Check sheet for the drawn part. Datum: minimum x, y, z corner. Units: mm. A direction names the side the tool comes from. Round coordinates to 2 decimals unless told otherwise and drop trailing zeros. Order: outer loops, then holes, each group sorted by start corner. A loop starts at its lowest first (then second) coordinate and runs counter-clockwise, first axis right, second up. Notation, with made-up numbers: (1.25, 1) -> (9.25, 1) arc R15 ccw to (9.25, 13) -> close; hole circle Ø2 at (34.5, 82). An arc over 180 degrees is marked (long way). Answer in a Markdown table with one row per item.
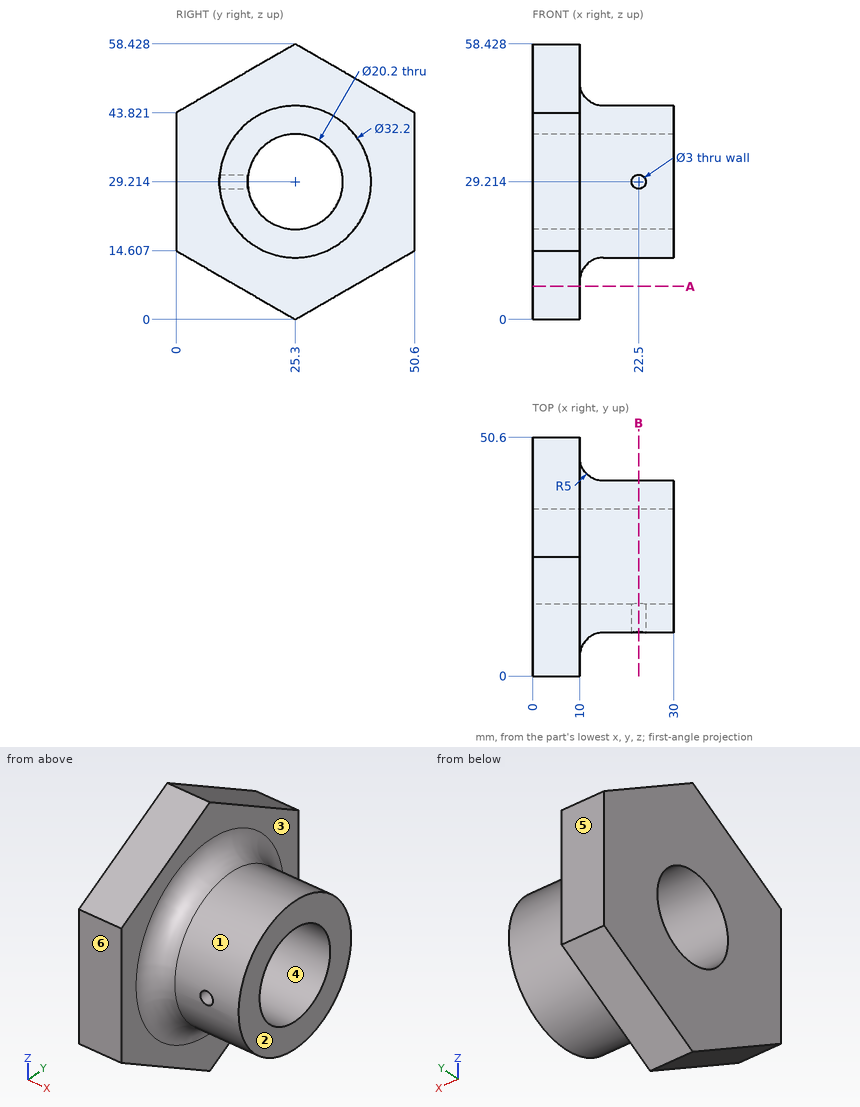
(1) Scan lines: probe 1 along Y at (x, z) = (22, 20.5); probe 2 along X at (y, z) = (36, 50); probe 3 along Y at (x, z) = (9, 36). Record each from-to range of solid material in increasing order. Write a range as from..to.
Solutions:
| item | result |
|---|---|
| probe 1 | 11.76..20.19, 30.41..38.84 |
| probe 2 | 0..10 |
| probe 3 | 0..17.82, 32.78..50.6 |
(2) Tool access check on the marked faces 1 and 2. Record the directions out of +Z, -Z, +X, -X, +Y, -Y that give a thin tool (end or side, any length) a straight path to the whole face; none if there is none.
Solutions:
| item | result |
|---|---|
| face 1 | +X |
| face 2 | +Z, -Z, +X, +Y, -Y |
(3) Draft check along Y on the marked faces 3, 4, 5 and 6. Enter one of: pulls with the +Y half, pulls with the -Y half, needs draft (parallel to the pull), parting line crosses it, or undercut.
Solutions:
| item | result |
|---|---|
| face 3 | needs draft |
| face 4 | undercut |
| face 5 | pulls with the +Y half |
| face 6 | pulls with the -Y half |
(4) Section check A-A on z = 7. Record the boundary of the cut face in (x, y), plus the area to 4 significant figures.
Solutions:
| item | result |
|---|---|
| outline | (0, 13.18) -> (10, 13.18) -> (10, 37.42) -> (0, 37.42) -> close |
| area | 242.5 mm^2 |
(5) Depth check by flat-ended pin: pin 1 Ø5 at (x, z) = (22.5, 29.21) entering from -Y; pin 2 Ø6 at (x, z) = (22.5, 31) entering from +Y; pin 3 Ø1 at (x, z) = (15.5, 23) entering from -Y. Enter the tip coordinate at first touch or a pass-through.
Solutions:
| item | result |
|---|---|
| pin 1 | y = 9.2 |
| pin 2 | y = 41.4 |
| pin 3 | y = 10.25 |
(6) Section check B-B on x = 22.5. Record the boundary of the cut face in (y, z), plus the area to 3 significant figures.
Solutions:
| item | result |
|---|---|
| outline | (9.27, 27.71) arc R16.1 ccw (long way) to (9.27, 30.71) -> (15.31, 30.71) arc R10.1 cw (long way) to (15.31, 27.71) -> close |
| area | 476 mm^2 |
